Study the drawing (mm; zero at the part's minimum x, y, z) and answer. A direction names the side the tool comes from. Coordinates: 2 decimals unless noted, no trailing zeros. Order: outer loops, then holes, each group sorted by start corner. A loop starts at its lowest first (then second) coordinate and runs counter-clockwise, first axis right, second up.
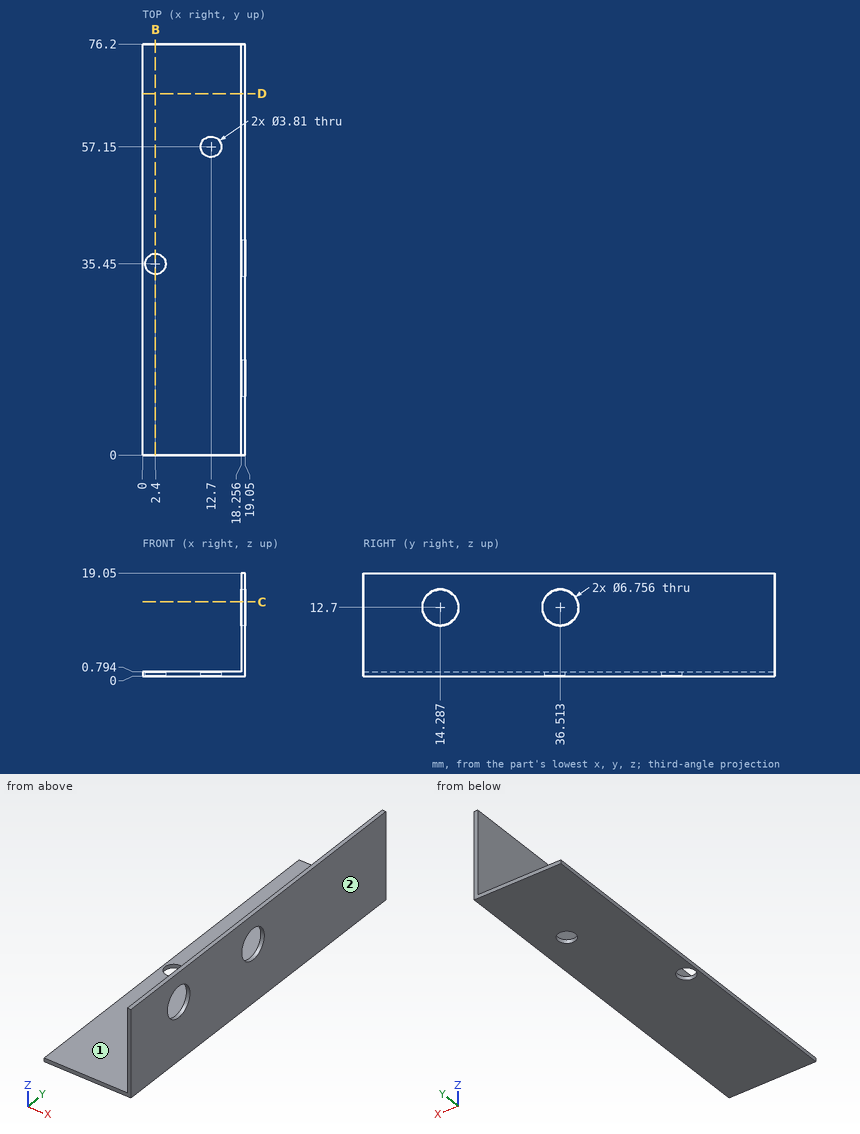
(1) Given pin 1 Ø2 at (x, y) = (5.5, 62) entering from +Z; pin 2 Ø1 at (y, z) = (41, 16.5) entering from -X, each flat-ended and moving along its own axis, determine where each tip first touches the part or whether it passes through.
(2) A tool of negligible diameter and unlimited length cuts with its end or side. For the marked faces 1 and 2, from which of +Z, -Z, +X, -X, +Y, -Y can it reach the whole face along a straight path? Write none if from no direction.
(3) Find the intervals of material crossed by probe 1 along Y at (x, z) = (12.7, 0.6) (1 decimal); probe 2 along Y at (x, z) = (2.4, 0.6) (1 decimal); probe 3 along X at (y, z) = (28.5, 17.25), in increasing order.
(4) Find section B-B on x = 2.4. Determine the outline of the cut face in (y, z) (1 decimal).
(5) Find section D-D on y = 67. Determine the outline of the cut face in (x, z).
(6) Find section C-C on z = 13.75. Determine the outline of the cut face in (x, y).
Resolved:
1. pin 1: stops at z = 0.79
1. pin 2: stops at x = 18.26
2. face 1: +Z, -X, +Y, -Y
2. face 2: +Z, -Z, +X, +Y, -Y
3. probe 1: y = 0 to 55.2, 59.1 to 76.2
3. probe 2: y = 0 to 33.5, 37.4 to 76.2
3. probe 3: x = 18.26 to 19.05
4. outline: (0, 0) - (33.5, 0) - (33.5, 0.8) - (0, 0.8) - close; (37.4, 0) - (76.2, 0) - (76.2, 0.8) - (37.4, 0.8) - close
5. outline: (0, 0) - (19.05, 0) - (19.05, 19.05) - (18.26, 19.05) - (18.26, 0.79) - (0, 0.79) - close
6. outline: (18.26, 0) - (19.05, 0) - (19.05, 11.08) - (18.26, 11.08) - close; (18.26, 17.5) - (19.05, 17.5) - (19.05, 33.3) - (18.26, 33.3) - close; (18.26, 39.72) - (19.05, 39.72) - (19.05, 76.2) - (18.26, 76.2) - close
